Verification items for this drawing (mm, ordinates from the low corner). Give positions to 0.01 mm unless a question says otherwise; leave off trailing zeros. Loops run counter-clockwise (first coordinate to the right, second up) from the corner with the lowest first, then second, coordinate; pieces in that order, holes last. Notation, with made-up numbers: M -34.5,67.25 L -8.5,67.25 A26 cw -8.5,96.25 Z; hole C 37,60.25 d10. An arc over 180 degrees is marked long. Put each result on its own line as item: value. Start each with the question number.
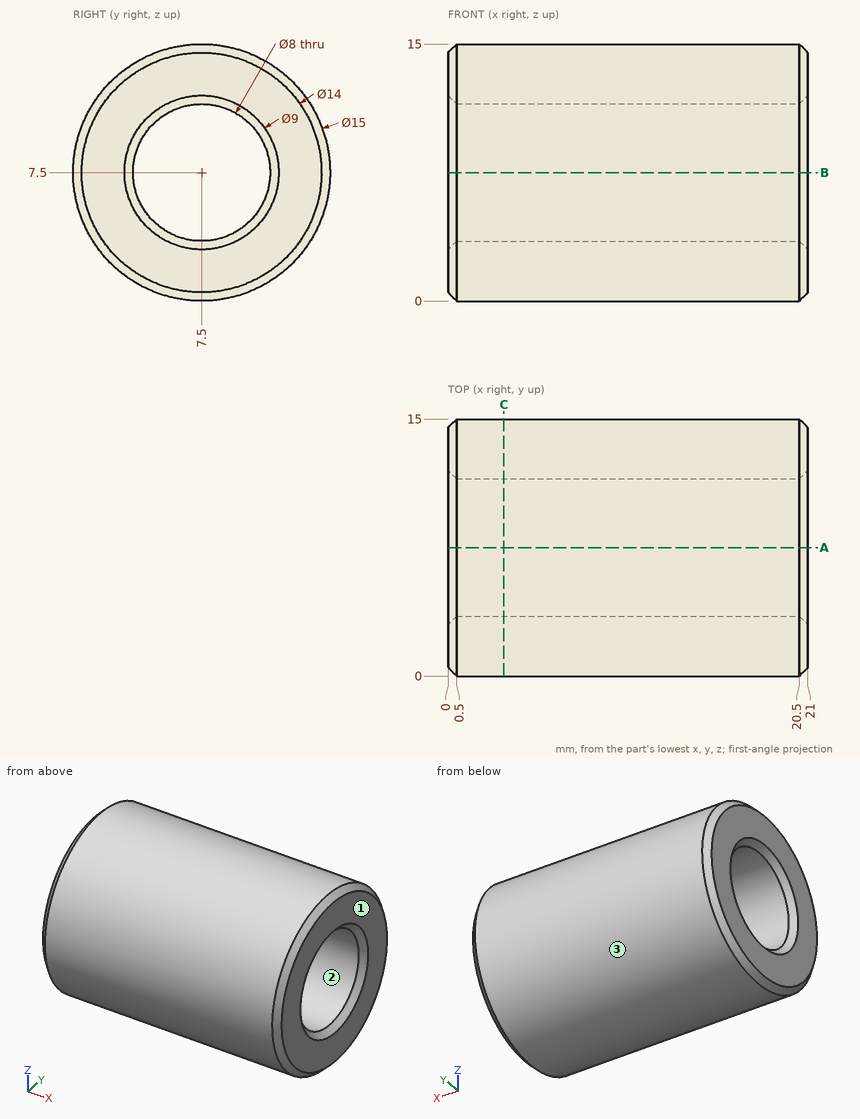
Q1. Go/stop test with flat-tipped pins: pin 1 (7 mm diameter, centred on y = 7.5, z = 7.5, fed in from +X); pin 2 (2 mm diameter, centred on x = 5.5, y = 13.5, fed in from +Z); pin 3 (2 mm diameter, centred on x = 4.5, z = 12, fed in from +Y); pin 4 (1.5 mm diameter, centred on x = 8.5, y = 9.5, fed in from +Z). Record where each tip stops, or that it passes through.
Q2. Scan lines: L1, parallel to Y at x = 6.75, z = 7.5; L2, parallel to Z at x = 1.75, y = 1.5; L3, parallel to Y at x = 6.5, z = 6. Record each from-to range of solid material in increasing order.
Q3. Release check for a two-part mould opening along Y. For the marked faces 1, 2 and 3 record: pulls with the +Y half, pulls with the -Y half, needs draft (parallel to the pull), parting line crosses it, or undercut.
Q4. Cross-section at C-C, the plane x = 3.25. Record the boundary of the cut face in (y, z), then the cut area to 3 significant figures.
Q5. Cross-section at A-A, the plane y = 7.5. Record the boundary of the cut face in (x, z), then the cut area to 3 significant figures.
Ans:
1. pin 1: passes through
1. pin 2: stops at z = 13.09
1. pin 3: stops at y = 14.13
1. pin 4: stops at z = 14.9
2. L1: y = 0 to 3.5, 11.5 to 15
2. L2: z = 3 to 12
2. L3: y = 0.15 to 3.79, 11.21 to 14.85
3. face 1: needs draft
3. face 2: undercut
3. face 3: parting line crosses it
4. outline: C 7.5,7.5 d15; hole C 7.5,7.5 d8
4. area: 126 mm^2
5. outline: M 0,0.5 L 0.5,0 L 20.5,0 L 21,0.5 L 21,3 L 20.5,3.5 L 0.5,3.5 L 0,3 Z; M 0,12 L 0.5,11.5 L 20.5,11.5 L 21,12 L 21,14.5 L 20.5,15 L 0.5,15 L 0,14.5 Z
5. area: 146 mm^2
